from build123d import *

# Parameters (mm, degrees)
ESQUISSE1_R             = 33
ESQUISSE1_R_2           = 32
BOSS_EXTRU_1_DEPTH      = 4
ESQUISSE2_R             = 33.6
ESQUISSE2_R_2           = 32
BOSS_EXTRU_2_DEPTH      = 4
ESQUISSE3_R             = 33
ESQUISSE3_R_2           = 32
BOSS_EXTRU_3_DEPTH      = 25.2
BOSS_EXTRU_4_DEPTH      = 12.5
BOSS_EXTRU_4_DEPTH_BACK = 64.2
ESQUISSE4_R             = 12.5
CONG_1_R                = 12.5
ESQUISSE5_W             = 1.5
ESQUISSE5_H             = 20.513996459
BOSS_EXTRU_5_DEPTH      = 18


with BuildPart() as part:
    # Esquisse1 → Boss.-Extru.1 (new body)
    with BuildSketch(Plane.XY):
        Circle(ESQUISSE1_R)
        Circle(ESQUISSE1_R_2, mode=Mode.SUBTRACT)
    extrude(amount=BOSS_EXTRU_1_DEPTH)

    # Esquisse2 → Boss.-Extru.2 (add)
    with BuildSketch(Plane.XY.offset(4)):
        Circle(ESQUISSE2_R)
        Circle(ESQUISSE2_R_2, mode=Mode.SUBTRACT)
    extrude(amount=BOSS_EXTRU_2_DEPTH)

    # Esquisse3 → Boss.-Extru.3 (add)
    with BuildSketch(Plane.XY.offset(8)):
        Circle(ESQUISSE3_R)
        Circle(ESQUISSE3_R_2, mode=Mode.SUBTRACT)
    extrude(amount=BOSS_EXTRU_3_DEPTH)



with BuildPart() as body_2:
    # Esquisse4 → Boss.-Extru.4 (new, two sides: drawn at the far end of the back side and taken through both)
    with BuildSketch(Plane(origin=(0, 0, 0), x_dir=(-1, 0, 0), z_dir=(0, 0, -1)).offset(-BOSS_EXTRU_4_DEPTH_BACK)):
        Circle(ESQUISSE4_R)
    extrude(amount=BOSS_EXTRU_4_DEPTH + BOSS_EXTRU_4_DEPTH_BACK)

    # Congé1
    cong_1_edges = [body_2.edges().sort_by_distance(p)[0] for p in [
        (12.5, 0, -12.5),
    ]]
    fillet(cong_1_edges, radius=CONG_1_R - 0.0001)  # a hair under: the kernel refuses the full size


with BuildPart() as part_1:
    add(part.part)

    add(body_2.part)  # Boss.-Extru.5 merges body 2
    # Esquisse5 → Boss.-Extru.5 (add)
    with BuildSketch(Plane.XY.offset(33.2)):
        with Locations((0, 22.734477942)):
            Rectangle(ESQUISSE5_W, ESQUISSE5_H)
        Polygon((28.196456473, -17.145257139), (10.430814407, -6.88825891), (11.180814407, -5.589220804), (28.946456473, -15.846219033), align=None)
        Polygon((-28.946456473, -15.846219033), (-11.180814407, -5.589220804), (-10.430814407, -6.88825891), (-28.196456473, -17.145257139), align=None)
    extrude(amount=-BOSS_EXTRU_5_DEPTH)


solid = part_1.part
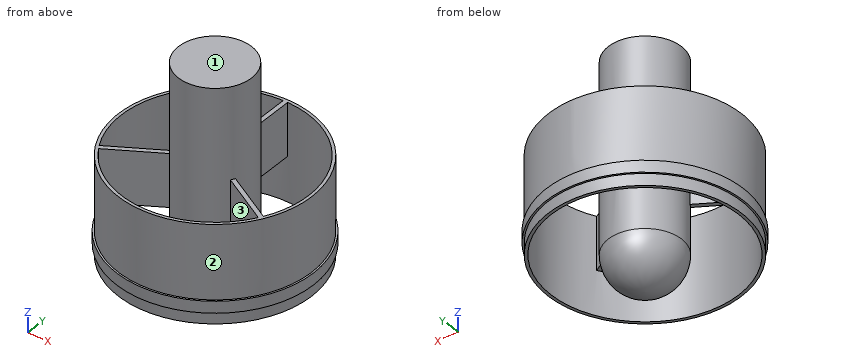
The model under review builds one solid part; all positions refer to its coordinate system, in mm. Face numbers are marked on the shaded views. Round coordinates to 2 decimals unless told otherwise and drop trailing zeros. Loops run counter-clockwise (first coordinate to the right, second up) from the corner with the lowest first, then second, coordinate; pieces in that order, holes last. Notation, with made-up numbers: (58, 76.25) -> (94, 76.25) arc R11 cw to (94, 85.25) -> close; hole circle Ø10 at (87.25, 13). An arc over 180 degrees is marked (long way). One line per question, with ' | ' between items. Start each with the question number.
Item 1: Add section C-C, the plane y = -26.5. Write out the cut boundary in (x, z), then the cut area to 3 significant figures.
Item 2: Add section A-A, the plane z = 12. Write out the cut boundary in (x, y).
Item 3: For pin 1 (9 mm diameter, centred on y = 21.5, z = 21.5, fed in from -X); pin 2 (9 mm diameter, centred on x = -16, y = -12, fed in from -Z); pin 3 (1.5 mm diameter, centred on x = -13, z = 33.5, fed in from +Y); pin 4 (2 mm diameter, centred on x = -16.5, y = -26, fed in from +Z), all flat-tipped, find the tip position at first contact; note any pin that passes through.
Item 4: Wall thickness on line 1 along Y through (x, z) = (0, 10); line 2 along Y through (x, z) = (0, 22); line 3 along X through (y, z) = (11.5, 21.5): over which ranges is each line inside the solid? List them lowest first. Write a range as [from, to].
Item 5: Draft analysis for pull direction Y (two halves, no side actions). For the marked faces 1, 2 and 3, state which applies: +Y half, -Y half, draft (parallel to the pull), parting line (faces both ways), or undercut.
Item 6: Add section D-D, the plane z = 46.5. Write out the cut boundary in (x, y), then the cut area to 3 significant figures.
Item 7: Add section B-B, the plane x = 18.5. Write out the cut boundary in (y, z), then the cut area to 3 significant figures.
Return value:
1) outline: (-20.66, 4) -> (-19.67, 4) -> (-19.67, 0) -> (-17.94, 0) -> (-17.94, 33.2) -> (-19.67, 33.2) -> (-19.67, 8) -> (-20.66, 8) -> close; (17.94, 0) -> (19.67, 0) -> (19.67, 4) -> (20.66, 4) -> (20.66, 8) -> (19.67, 8) -> (19.67, 33.2) -> (17.94, 33.2) -> close | area: 123 mm2
2) outline: circle Ø66 at (0, 0); circle Ø25 at (0, 0); hole circle Ø64 at (0, 0)
3) pin 1: stops at x = -28.28 | pin 2: stops at z = 15.2 | pin 3: stops at y = 30.62 | pin 4: passes through
4) line 1: y = [-33, -32], [-12.5, 12.5], [32, 33] | line 2: y = [-33, -32], [-12.5, 33] | line 3: x = [-30.93, -29.86], [-4.9, 4.9], [29.86, 30.93]
5) face 1: draft | face 2: parting line | face 3: undercut
6) outline: circle Ø25 at (0, 0) | area: 491 mm2
7) outline: (-28.05, 4) -> (-27.33, 4) -> (-27.33, 0) -> (-26.11, 0) -> (-26.11, 33.2) -> (-27.33, 33.2) -> (-27.33, 8) -> (-28.05, 8) -> close; (-11.55, 15.2) -> (-9.81, 15.2) -> (-9.81, 33.2) -> (-11.55, 33.2) -> close; (26.11, 0) -> (27.33, 0) -> (27.33, 4) -> (28.05, 4) -> (28.05, 8) -> (27.33, 8) -> (27.33, 33.2) -> (26.11, 33.2) -> close | area: 118 mm2
